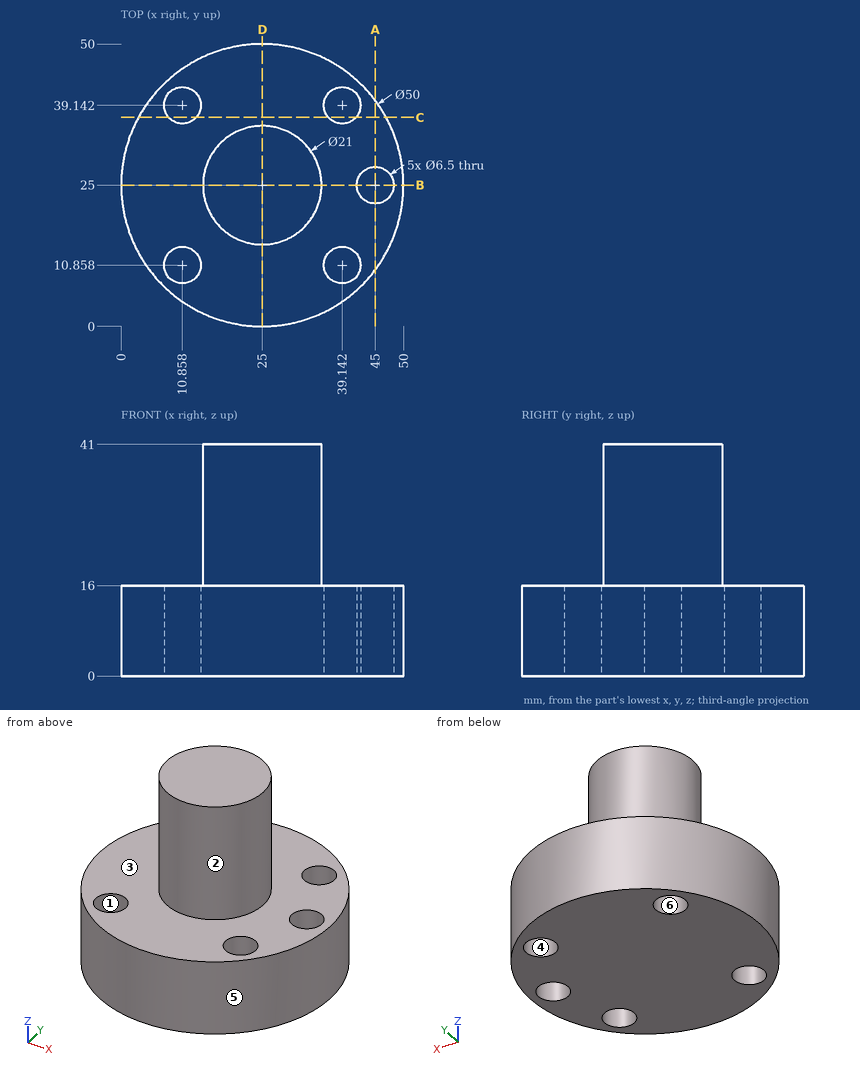
The figure shows three views and two pictorial views of one solid part (mm, origin at its lowest corner). Answer the questions. A direction names the side the tool comes from. Give positions to 0.01 mm unless a question says otherwise; leave off trailing zeros. Write each loop counter-clockwise with the first axis right and the second up, starting at its lowest first coordinate (ties: lowest second). Pieces come first, ordered by that corner, then holes.
Q1. The part is cut by section C-C on y = 37. Give the vertices of the cut face in (x, z), and give its area (3 significant figures).
Answer:
outline: (3.07, 0) - (8.41, 0) - (8.41, 16) - (3.07, 16) - close; (13.3, 0) - (36.7, 0) - (36.7, 16) - (13.3, 16) - close; (41.59, 0) - (46.93, 0) - (46.93, 16) - (41.59, 16) - close
area: 545 mm2
Q2. The part is cut by section B-B on y = 25. Give the vertices of the cut face in (x, z).
Answer:
outline: (0, 0) - (41.75, 0) - (41.75, 16) - (35.5, 16) - (35.5, 41) - (14.5, 41) - (14.5, 16) - (0, 16) - close; (48.25, 0) - (50, 0) - (50, 16) - (48.25, 16) - close
Q3. The part is cut by section A-A on x = 45. Give the vertices of the cut face in (y, z), and give its area (3 significant figures).
Answer:
outline: (10, 0) - (21.75, 0) - (21.75, 16) - (10, 16) - close; (28.25, 0) - (40, 0) - (40, 16) - (28.25, 16) - close
area: 376 mm2
Q4. The part is cut by section D-D on x = 25. Give the vertices of the cut face in (y, z).
Answer:
outline: (0, 0) - (50, 0) - (50, 16) - (35.5, 16) - (35.5, 41) - (14.5, 41) - (14.5, 16) - (0, 16) - close
Q5. Given pin 1 (5 mm diameter, centred on x = 10.86, y = 39.14, fed in from -Z); pin 2 (6 mm diameter, centred on y = 37, z = 31.5, fed in from -X); pin 3 (12 mm diameter, centred on x = 17, y = 44.5, fed in from +Z); pin 4 (3 mm diameter, centred on y = 29.5, z = 21.5, fed in from +X), each flat-ended and moving along its own axis, determine where each tip first touches the part or whether it passes through.
Answer:
pin 1: passes through
pin 2: stops at x = 19.59
pin 3: stops at z = 16
pin 4: stops at x = 35.06
Q6. For a pull along X with two mould halves and no side action, classify the marked faces 3, 4, 5 and 6 as released by +X, released by -X, zero draft, split by the parting line, or undercut.
Answer:
face 3: zero draft
face 4: undercut
face 5: split by the parting line
face 6: undercut
Q7. Straight lines are drawn through the part: L1, parallel to X at y = 12.5, z = 6.5; L2, parallel to X at y = 10.5, z = 10 (1 decimal); L3, parallel to Z at x = 27.5, y = 3. For each, find the intervals that lie inside material, in ascending order.
Answer:
L1: x = 3.35 to 8.05, 13.66 to 36.34, 41.95 to 46.65
L2: x = 4.6 to 7.6, 14.1 to 35.9, 42.4 to 45.4
L3: z = 0 to 16
Q8. A tool of negligible diameter and unlimited length cuts with its end or side. For the marked faces 1 and 2, from which of +Z, -Z, +X, -X, +Y, -Y can it reach the whole face along a straight path? Write none if from no direction.
Answer:
face 1: +Z, -Z
face 2: +Z
